```python
from build123d import *

# Parameters (mm, degrees)
ESBO_O1_W                = 90
ESBO_O1_H                = 110
RESSALTO_EXTRUS_O1_DEPTH = 3
ESBO_O2_W                = 50
ESBO_O2_H                = 39.951487405
CORTE_EXTRUS_O2_DEPTH    = 143.158362399
ESBO_O4_W                = 90
ESBO_O4_H                = 75
RESSALTO_EXTRUS_O2_DEPTH = 5
ESBO_O5_W                = 90
ESBO_O5_H                = 75
RESSALTO_EXTRUS_O3_DEPTH = 3
FILETE5_R                = 1


with BuildPart() as part:
    # Esboço1 → Ressalto-extrusão1 (new body)
    with BuildSketch(Plane(origin=(0, 0, 0), x_dir=(1, 0, 0), z_dir=(0, 1, 0))):
        with Locations((45, 55)):
            Rectangle(ESBO_O1_W, ESBO_O1_H)
    extrude(amount=RESSALTO_EXTRUS_O1_DEPTH)

    # Esboço2 → Corte-extrusão2 (cut, through all)
    with BuildSketch(Plane(origin=(0, 3, 0), x_dir=(1, 0, 0), z_dir=(0, 1, 0))):
        with Locations((45, 19.975743703)):
            Rectangle(ESBO_O2_W, ESBO_O2_H)
    extrude(amount=-CORTE_EXTRUS_O2_DEPTH, mode=Mode.SUBTRACT)

    # Esboço4 → Ressalto-extrusão2 (add)
    with BuildSketch(Plane.XY):
        with Locations((45, 37.5)):
            Rectangle(ESBO_O4_W, ESBO_O4_H)
    extrude(amount=RESSALTO_EXTRUS_O2_DEPTH)

    # Esboço5 → Ressalto-extrusão3 (add)
    with BuildSketch(Plane(origin=(0, 0, -110), x_dir=(-1, 0, 0), z_dir=(0, 0, -1))):
        with Locations((-45, 37.5)):
            Rectangle(ESBO_O5_W, ESBO_O5_H)
    extrude(amount=RESSALTO_EXTRUS_O3_DEPTH)

    # Filete5
    filete5_edges = [part.edges().sort_by_distance(p)[0] for p in [
        (45, 0, 5),
        (45, 0, -113),
    ]]
    fillet(filete5_edges, radius=FILETE5_R)


solid = part.part
```
Model file for the job. Use its own axes, mm. A direction names the side the tool comes from. Coordinates: 2 decimals unless noted, no trailing zeros. Write each loop counter-clockwise with the first axis right and the second up, starting at its lowest first coordinate (ties: lowest second). Pieces come first, ordered by that corner, then holes. Notation, with made-up numbers: (-26.5, 34.5) - (14.5, 34.5) arc R12 ccw to (14.5, 43.5) - close; hole circle Ø11 at (74.5, -24). An arc over 180 degrees is marked (long way). One line per question, with ' | ' between items. Start each with the question number.
Q1. Cut at B-B, the plane x = 48.5. List the corners of the cut face in (y, z), then the cut area to 3 significant figures.
Q2. Pull direction X, two halves, no side cores. Call faces 1 (the face through (46, 0, -66)), 2 (the face through (45, 2, -39.951)), 3 (the face through (90, 1, -54)): pulls with the +X half, pulls with the -X half, needs draft (parallel to the pull), parting line crosses it, or undercut.
Q3. Drill centre lines: line 1 (Z direction, x = 72, y = 33.5); line 2 (Y direction, x = 58, z = -80.5). Where is each one in solid material? Low to high. Write a range as [from, to].
Q4. Cut at A-A, the plane y = 65. List the corners of the cut face in (x, z), then the cut area to 3 significant figures.
Q5. Cut at C-C, the plane z = -13. List the corners of the cut face in (x, y).
Q6. Cut at D-D, the plane x = 9.5. List the corners of the cut face in (y, z).
Q7. 3-axis set-ups, long thin cutter, end or side, ignore diameter. For faces 4 (the face through (0, 1, -54)), 5 (the face through (46, 40, -110)), 6 (the face through (20, 2, -20)): which of +Z, -Z, +X, -X, +Y, -Y reach the whole face in a straight line?
Q8. Pin check, flat tips, straight feed: pin 1 (2 mm diameter, centred on x = 46.5, z = -81, fed in from +Y); pin 2 (12 mm diameter, centred on x = 22, z = -7.5, fed in from -Y); pin 3 (12 mm diameter, centred on x = 38.5, z = -11.5, fed in from +Y). Stop position of each tip, or through.
Answer below:
1) outline: (0, -112) arc R1 ccw to (1, -113) - (75, -113) - (75, -110) - (3, -110) - (3, -39.95) - (0, -39.95) - close; (0, 0) - (75, 0) - (75, 5) - (1, 5) arc R1 ccw to (0, 4) - close | area: 810 mm^2
2) face 1: needs draft | face 2: undercut | face 3: pulls with the +X half
3) line 1: [-113, -110], [0, 5] | line 2: [0, 3]
4) outline: (0, -113) - (90, -113) - (90, -110) - (0, -110) - close; (0, 0) - (90, 0) - (90, 5) - (0, 5) - close | area: 720 mm^2
5) outline: (0, 0) - (20, 0) - (20, 3) - (0, 3) - close; (70, 0) - (90, 0) - (90, 3) - (70, 3) - close
6) outline: (0, -112) arc R1 ccw to (1, -113) - (75, -113) - (75, -110) - (3, -110) - (3, 0) - (75, 0) - (75, 5) - (1, 5) arc R1 ccw to (0, 4) - close
7) face 4: +Z, -Z, -X, +Y, -Y | face 5: +X, -X, +Y | face 6: +Y, -Y
8) pin 1: y = 3 | pin 2: y = 0 | pin 3: through
